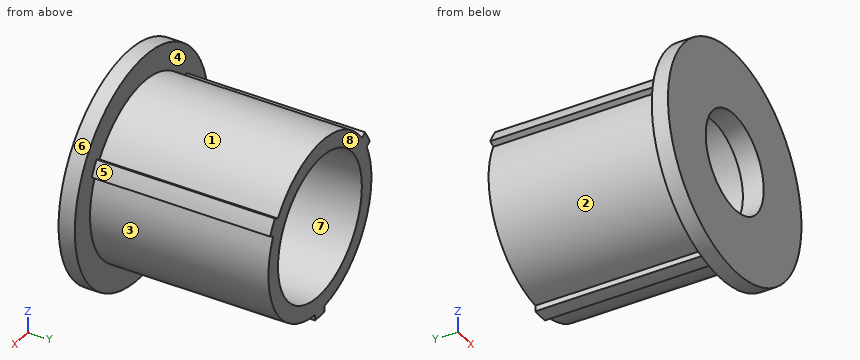
from build123d import *

# Parameters (mm, degrees)
BOSS_EXTRUDE1_DEPTH = 19.05
SKETCH6_W           = 0.608326788
SKETCH6_H           = 1.5875
SKETCH8_W           = 2.576826788
SKETCH8_H           = 1.5875
SKETCH12_R          = 6.985
CUT_EXTRUDE7_DEPTH  = 17.018
SKETCH13_R          = 4.826
CUT_EXTRUDE8_DEPTH  = 20.05


with BuildPart() as part:
    # Sketch1 → Boss-Extrude1 (new body)
    with BuildSketch(Plane(origin=(0, 0, 0), x_dir=(1, 0, 0), z_dir=(0, 1, 0))):
        with BuildLine():
            Line((-0.79375, 9.109483901), (-0.79375, 8.535673212))
            ThreePointArc((-0.79375, 8.535673212), (-7.424002774, 4.28625), (-7.78898484, -3.580428942))
            Line((-7.78898484, -3.580428942), (-8.285919473, -3.867334286))
            ThreePointArc((-8.285919473, -3.867334286), (-7.918936292, -4.572), (-7.492169473, -5.242149615))
            Line((-7.492169473, -5.242149615), (-6.99523484, -4.95524427))
            ThreePointArc((-6.99523484, -4.95524427), (0, -8.5725), (6.99523484, -4.95524427))
            Line((6.99523484, -4.95524427), (7.492169473, -5.242149615))
            ThreePointArc((7.492169473, -5.242149615), (7.918936292, -4.572), (8.285919473, -3.867334286))
            Line((8.285919473, -3.867334286), (7.78898484, -3.580428942))
            ThreePointArc((7.78898484, -3.580428942), (7.424002774, 4.28625), (0.79375, 8.535673212))
            Line((0.79375, 8.535673212), (0.79375, 9.109483901))
            ThreePointArc((0.79375, 9.109483901), (0, 9.144), (-0.79375, 9.109483901))
        make_face()
    extrude(amount=BOSS_EXTRUDE1_DEPTH)

    # Sketch6 → Cut-Revolve2 (revolve, cut)
    with BuildSketch(Plane(origin=(0, 0, 0), x_dir=(0, 0, -1), z_dir=(1, 0, 0))):
        with Locations((8.839836606, 0.79375)):
            Rectangle(SKETCH6_W, SKETCH6_H)
    revolve(axis=Axis((0, 19.730213777, 0), (0, -1, 0)), mode=Mode.SUBTRACT)

    # Sketch8 → Revolve2 (revolve)
    with BuildSketch(Plane(origin=(0, 0, 0), x_dir=(0, 0, -1), z_dir=(1, 0, 0))):
        with Locations((9.824086606, 0.79375)):
            Rectangle(SKETCH8_W, SKETCH8_H)
    revolve(axis=Axis((0, 4.48386458, 0), (0, -1, 0)))

    # Sketch12 → Cut-Extrude7 (cut)
    with BuildSketch(Plane(origin=(0, 19.05, 0), x_dir=(1, 0, 0), z_dir=(0, 1, 0))):
        Circle(SKETCH12_R)
    extrude(amount=-CUT_EXTRUDE7_DEPTH, mode=Mode.SUBTRACT)

    # Sketch13 → Cut-Extrude8 (cut, through all)
    with BuildSketch(Plane.XZ):
        Circle(SKETCH13_R)
    extrude(amount=-CUT_EXTRUDE8_DEPTH, mode=Mode.SUBTRACT)


solid = part.part
The listing builds one solid part. Answer for the finished solid, in the listing's coordinates (mm). Face numbers are marked on the shaded views. A direction names the side the tool comes from. Round coordinates to 2 decimals unless told otherwise and drop trailing zeros. Write each loop counter-clockwise with the first axis right and the second up, starting at its lowest first coordinate (ties: lowest second). Pieces come first, ordered by that corner, then holes. Notation, with made-up numbers: M 37.25,8.5 L 57.25,8.5 A36 cw 57.25,46.5 Z; hole C 79.25,45.25 d8. An arc over 180 degrees is marked long. Write each question's results on one line, items separated by ' | '. Start each with the question number.
Item 1: Straight lines are drawn through the part: L1, parallel to Z at x = 0, y = 6 (1 decimal); L2, parallel to X at y = 6, z = 0 (1 decimal); L3, parallel to X at y = 7, z = -9. For each, find the intervals that lie inside material, in ascending order. Write a range as [from, to].
Item 2: Flat-ended cylindrical pins translate along their axes: pin 1 Ø1 at (x, y) = (-5.5, 16) entering from +Z; pin 2 Ø6 at (x, y) = (8.5, 5) entering from -Z; pin 3 Ø6 at (x, y) = (9, 15.5) entering from -Z; pin 4 Ø11 at (x, z) = (-2.5, 3) entering from +Y. Find the tip coordinate at first contact, or state that the pin passes through.
Item 3: For the marked faces 1, 2, 3, 4 and 5, determine the directions among +Z, -Z, +X, -X, +Y, -Y from which every point of the face is accessible in a straight line to the end or side of a thin tool.
Item 4: A cutting plane is placed at C-C on y = 4.5. Write down the section's boundary in (x, z) (1 decimal), and give its area (3 significant figures).
Item 5: For a pull along X with two mould halves and no side action, classify the marked faces 6, 7 and 8 as pulls with the +X half, pulls with the -X half, needs draft (parallel to the pull), parting line crosses it, or undercut.
Item 6: A cutting plane is placed at D-D on z = 10.25. Write down the section's boundary in (x, y), and give its area (3 significant figures).
Check sheet entries:
1) L1: [-9.1, -7], [7, 8.6] | L2: [-8.6, -7], [7, 8.6] | L3: [-0.79, 0.79]
2) pin 1: z = 6.96 | pin 2: z = -6.58 | pin 3: z = -6.12 | pin 4: y = 19.05
3) face 1: +Z, +Y | face 2: -X, +Y | face 3: +X, +Y | face 4: +Y | face 5: +Z, +X, +Y
4) outline: M -8.3,3.9 L -7.8,3.6 A8.6 ccw -0.8,-8.5 L -0.8,-9.1 A9.1 ccw 0.8,-9.1 L 0.8,-8.5 A8.6 ccw 7.8,3.6 L 8.3,3.9 A9.1 ccw 7.5,5.2 L 7,5 A8.6 ccw -7,5 L -7.5,5.2 A9.1 ccw Z; hole C 0,0 d14 | area: 80.3 mm²
5) face 6: parting line crosses it | face 7: undercut | face 8: needs draft
6) outline: M -4.29,0 L 4.29,0 L 4.29,1.59 L -4.29,1.59 Z | area: 13.6 mm²
